Geometry: see drawing. Coordinates: mm, zero at the bounding-box minimum. A direction names the side the tool comes from. Give positions to 0.01 mm unless a question says otherwise; leave off trailing zeros. Loops run counter-clockwise (first coordinate to the right, second up) from the corner with the lowest first, then second, coordinate; pieces in that order, holes last. Notation, with made-up numbers: (-9.75, 80) -> (16.25, 80) arc R8 cw to (16.25, 90) -> close; hole circle Ø10 at (-18.5, 54.5). An arc over 180 degrees is marked (long way). Return JSON: item names as keys, results as strings. Group by question number.
(1) Access query for the marked faces 1 and 2. Directions: +Z, -Z, +X, -X, +Y, -Y. A direction counts if a zero-diameter tool reaches every point of the face in a straight line with its end or side. Return the directions, or none.
(2) Cut plane C-C on z = 2.75. Give the number of separate pieces and of enclosed holes in the cut face.
(3) Draft query along X for the marked faces 3, 4 and 5. Return one class per face: released by +X, released by -X, zero draft, split by the parting line, or undercut.
(4) Ray query, line 1 (X direction, y = 10, z = 1.1) (1 decimal); line 2 (Z direction, x = 10, y = 12.25). Return the intervals inside material, ascending. Write a range as from..to.
(5) Cut plane A-A on z = 3.75. Return loops of the section in (x, y) (1 decimal).
(6) Pin query (flat end, axial travel): pin 1 (0.8 mm diameter, centred on y = 5.5, z = 5, fed in from +X) (3 decimals); pin 2 (1.5 mm diameter, centred on y = 13, z = 4.5, fed in from +X) (3 decimals); pin 3 (3 mm diameter, centred on x = 7.5, y = 5, fed in from +Z). Return the tip coordinate at first contact, or that it passes through.
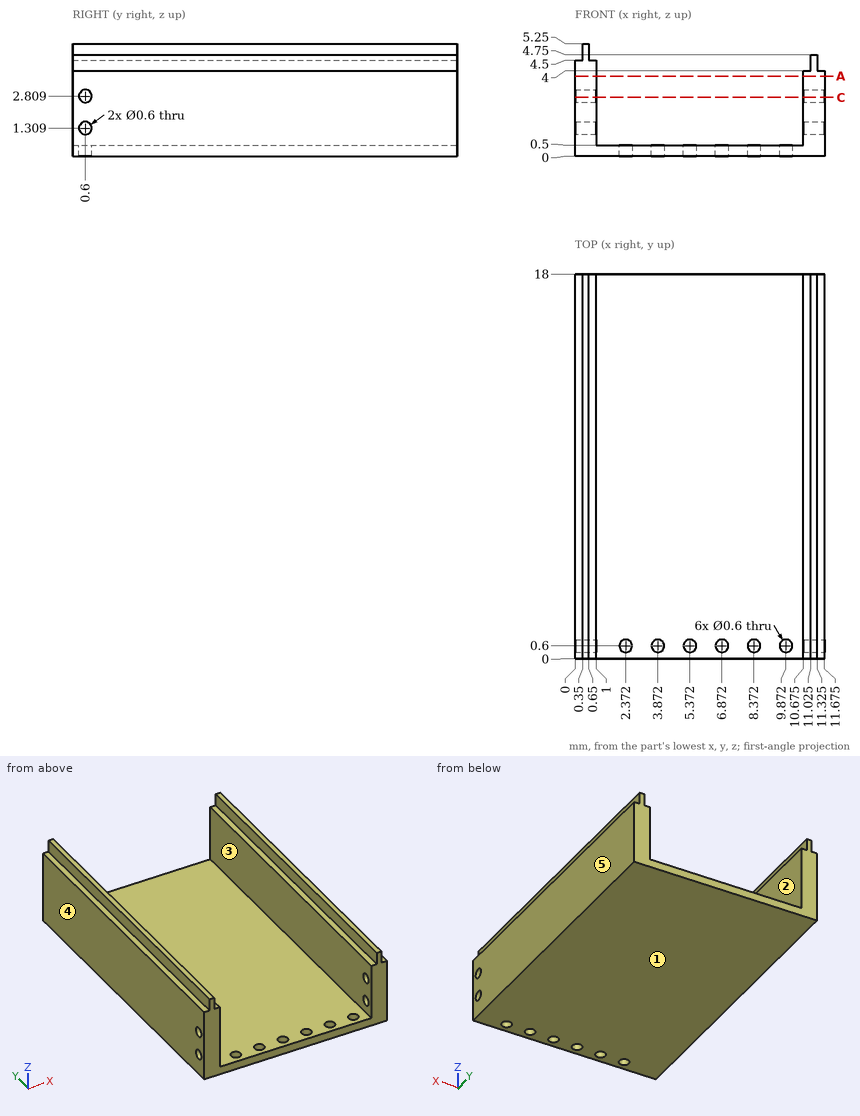
Answers:
{
 "1": {"face 1": "-Z, +X, -X, +Y, -Y", "face 2": "+Z, +Y, -Y"},
 "2": {"separate pieces": "4", "enclosed holes": "0"},
 "3": {"face 3": "undercut", "face 4": "released by -X", "face 5": "released by +X"},
 "4": {"line 1": "0..1, 10.7..11.7", "line 2": "0..0.5"},
 "5": {"outline": "(0, 0) -> (1, 0) -> (1, 18) -> (0, 18) -> close; (10.7, 0) -> (11.7, 0) -> (11.7, 18) -> (10.7, 18) -> close"},
 "6": {"pin 1": "x = 11.325", "pin 2": "x = 11.675", "pin 3": "z = 0.5"}
}
